from build123d import *

# Parameters (mm, degrees)
SKETCH1_R           = 2.1
BOSS_EXTRUDE1_DEPTH = 5
FILLET1_R           = 3


with BuildPart() as part:
    # Sketch1 → Boss-Extrude1 (new body)
    with BuildSketch(Plane(origin=(0, 0, 0), x_dir=(1, 0, 0), z_dir=(0, 1, 0))):
        with BuildLine():
            Line((72, -9.503100502), (72, -4.5))
            ThreePointArc((72, -4.5), (75.181980515, 3.181980515), (67.5, 0))
            Line((67.5, 0), (67.5, -8.236120217))
            ThreePointArc((67.5, -8.236120217), (35.23528273, -6.295142783), (4.5, -16.301229399))
            Line((4.5, -16.301229399), (4.5, 0))
            ThreePointArc((4.5, 0), (1.722075446, 4.157457896), (-3.181980515, 3.181980515))
            Line((-3.181980515, 3.181980515), (-3.181980515, -3.181980515))
            ThreePointArc((-3.181980515, -3.181980515), (-1.722075446, -4.157457896), (0, -4.5))
            Line((0, -4.5), (0, -22.629109119))
            Line((0, -22.629109119), (4.5, -22.629109119))
            ThreePointArc((4.5, -22.629109119), (46.093164739, -11.519039327), (87.727526709, -22.473714454))
            Line((87.727526709, -22.473714454), (87.727526709, -16.152250539))
            ThreePointArc((87.727526709, -16.152250539), (80.027772069, -12.439738504), (72, -9.503100502))
        make_face()
        with Locations(Location((0, 0, 0), (0, 0, 270))):
            Circle(SKETCH1_R, mode=Mode.SUBTRACT)
        with Locations(Location((72, 0, 0), (0, 0, 270))):
            Circle(SKETCH1_R, mode=Mode.SUBTRACT)
    extrude(amount=BOSS_EXTRUDE1_DEPTH)

    # Fillet1
    fillet1_edges = [part.edges().sort_by_distance(p)[0] for p in [
        (-3.181980515, 2.5, 3.181980515),
        (-3.181980515, 2.5, -3.181980515),
        (4.5, 2.5, 16.301229399),
        (67.5, 2.5, 8.236120217),
        (72, 2.5, 4.5),
        (72, 2.5, 9.503100502),
        (87.727526709, 2.5, 16.152250539),
        (4.5, 2.5, 22.629109119),
        (0, 2.5, 22.629109119),
    ]]
    fillet(fillet1_edges, radius=FILLET1_R)


solid = part.part
Part model, mm, in its own coordinate system. A direction names the side the tool comes from. Give positions to 0.01 mm unless a question says otherwise; leave off trailing zeros. Write each loop counter-clockwise with the first axis right and the second up, starting at its lowest first coordinate (ties: lowest second). Pieces come first, ordered by that corner, then holes.
1) Cut at C-C on x = 46. Write the cut outline in (y, z).
Resolved:
outline: (0, 5.59) - (5, 5.59) - (5, 11.52) - (0, 11.52) - close
2) Which spindle directions (+Z, -Z, +X, -X, +Y, -Y) get a long thin tool onto all of the face, cutting with end or side? Do faces 1 (the face through (80.254, 2.465, 12.536)), 2 (the face through (0, 2, 12)), 3 (the face through (4.5, 2, 6)), 4 (the face through (42, 5, 11)). Say none if no direction does.
Resolved:
face 1: +X, +Y, -Y
face 2: +Z, -X, +Y, -Y
face 3: -Z, +Y, -Y
face 4: +Z, -Z, +X, -X, +Y
3) Pin check, flat tips, straight feed: pin 1 (1 mm diameter, centred on y = 4, z = 6.5, fed in from +X); pin 2 (3 mm diameter, centred on x = 34.5, y = 3.5, fed in from +Z); pin 3 (1.3 mm diameter, centred on y = 2.5, z = 3.5, fed in from -X). Stop position of each tip, or through.
Resolved:
pin 1: stops at x = 72.13
pin 2: stops at z = 12.57
pin 3: stops at x = -2.86
4) Cut at A-A on y = 1.65. Write the cut outline in (x, z), then the cut area to 3 significant figures.
Resolved:
outline: (-3.18, -1.49) arc R3 ccw to (-0.55, -4.47) arc R4.5 ccw to (4.5, 0) - (4.5, 11.39) arc R3 cw to (8.8, 14.1) arc R86.74 ccw to (63.89, 7.41) arc R3 cw to (67.5, 4.47) - (67.5, 0) arc R4.5 ccw (long way) to (73.8, 4.12) arc R3 cw to (72, 6.87) - (72, 7.32) arc R3 cw to (74.04, 10.16) arc R86.74 ccw to (86.11, 15.29) arc R3 ccw to (87.73, 17.96) - (87.73, 22.47) arc R84 cw to (5.18, 22.25) arc R3 ccw to (3.71, 22.63) - (3, 22.63) arc R3 ccw to (0, 19.63) - (0, 4.5) arc R4.5 ccw to (-0.55, 4.47) arc R3 ccw to (-3.18, 1.49) - close; hole circle Ø4.2 at (0, 0); hole circle Ø4.2 at (72, 0)
area: 714 mm2
5) Probe L1, parallel to X at y = 2, z = 0; L2, parallel to X at y = 1.7, z = -1.5; L3, parallel to X at y = 0.5, z = 19.5. List the from-to ranges inside material, lowest first.
Resolved:
L1: x = -3.18 to -2.1, 2.1 to 4.5, 67.5 to 69.9, 74.1 to 76.5
L2: x = -3.18 to -1.47, 1.47 to 4.24, 67.76 to 70.53, 73.47 to 76.24
L3: x = 0 to 10.51, 81.99 to 87.73
6) Cut at B-B on x = 30.5. Write the cut outline in (y, z).
Resolved:
outline: (0, 7.03) - (5, 7.03) - (5, 13.01) - (0, 13.01) - close
7) Two-plate mould, pull along Z, no slides. Class faces 5 (the face through (0.9, 2.54, 21.77)), 6 (the face through (74.577, 2.465, -3.689)), 7 (the face through (66.422, 2.535, 6.772)), 8 (the face through (42, 0, 11)): released by +Z, released by -Z, zero draft, split by the parting line, or undercut.
Resolved:
face 5: released by +Z
face 6: undercut
face 7: released by -Z
face 8: zero draft
